```python
from build123d import *

# Parameters (mm, degrees)
SKETCH3_W                = 25.4
SKETCH3_H                = 25.4
SKETCH3_W_2              = 21.336
SKETCH3_H_2              = 21.336
BOSS_EXTRUDE1_DEPTH      = 1219.2
BOSS_EXTRUDE1_DEPTH_BACK = 1219.2
FILLET1_R                = 3.175
FILLET2_R                = 1.5875


with BuildPart() as part:
    # Sketch3 → Boss-Extrude1 (new body, two sides)
    with BuildSketch(Plane.XY) as boss_extrude1_sk:
        Rectangle(SKETCH3_W, SKETCH3_H)
        Rectangle(SKETCH3_W_2, SKETCH3_H_2, mode=Mode.SUBTRACT)
    extrude(amount=BOSS_EXTRUDE1_DEPTH)
    extrude(boss_extrude1_sk.sketch, amount=-BOSS_EXTRUDE1_DEPTH_BACK)

    # Fillet1
    fillet1_edges = [part.edges().sort_by_distance(p)[0] for p in [
        (12.7, -12.7, 0),
        (-12.7, -12.7, 0),
        (-12.7, 12.7, 0),
        (12.7, 12.7, 0),
    ]]
    fillet(fillet1_edges, radius=FILLET1_R)

    # Fillet2
    fillet2_edges = [part.edges().sort_by_distance(p)[0] for p in [
        (10.668, -10.668, 0),
        (10.668, 10.668, 0),
        (-10.668, 10.668, 0),
        (-10.668, -10.668, 0),
    ]]
    fillet(fillet2_edges, radius=FILLET2_R)


solid = part.part
```
Build history of the part. All positions in model axes, mm. Give positions to 0.01 mm unless a question says otherwise; leave off trailing zeros. Order: outer loops, then holes, each group sorted by start corner. A loop starts at its lowest first (then second) coordinate and runs counter-clockwise, first axis right, second up. Notation, with made-up numbers: M -8,37 L 40,37 A19 cw 40,71 Z; hole C 63,-9.75 d2. An arc over 180 degrees is marked long. Return JSON: item names as keys, results as strings.
Q1. Band-saw the part on A-A (y = -0.25). Give the cut face in (x, z), then the cut area to 3 significant figures.
Answer list:
{"outline": "M -12.7,-1219.2 L -10.67,-1219.2 L -10.67,1219.2 L -12.7,1219.2 Z; M 10.67,-1219.2 L 12.7,-1219.2 L 12.7,1219.2 L 10.67,1219.2 Z", "area": "9,910 mm^2"}
Q2. Wall check: probe 1 along X at (y, z) = (-7.25, 604.5); probe 2 along X at (y, z) = (9.75, 588). Give the ranges that are in metal, low to high. Write a range as from..to.
Answer list:
{"probe 1": "x = -12.7..-10.67, 10.67..12.7", "probe 2": "x = -12.69..-10.52, 10.52..12.69"}
